from build123d import *

# Parameters (mm, degrees)
SKETCH_1_W          = 35
SKETCH_1_H          = 35
EXTRUDE_1_DEPTH     = 45
SKETCH_2_R          = 8.5
EXTRUDE_2_DEPTH     = 2.8
SKETCH_4_W          = 24
SKETCH_4_H          = 24
CUT_EXTRUDE_1_DEPTH = 40
SKETCH_5_R          = 3.25
CUT_EXTRUDE_2_DEPTH = 62.774509306


with BuildPart() as part:
    # 草图1 → 凸台-拉伸1 (new body)
    with BuildSketch(Plane(origin=(0, 0, 0), x_dir=(1, 0, 0), z_dir=(0, 1, 0))):
        Rectangle(SKETCH_1_W, SKETCH_1_H)
    extrude(amount=EXTRUDE_1_DEPTH)

    # 草图2 → 凸台-拉伸2 (add)
    with BuildSketch(Plane(origin=(0, 45, 0), x_dir=(1, 0, 0), z_dir=(0, 1, 0))):
        with Locations(Location((0, 0, 0), (0, 0, 270))):
            Circle(SKETCH_2_R)
    extrude(amount=EXTRUDE_2_DEPTH)

    # 草图4 → 切除-拉伸1 (cut)
    with BuildSketch(Plane.XZ):
        Rectangle(SKETCH_4_W, SKETCH_4_H)
    extrude(amount=-CUT_EXTRUDE_1_DEPTH, mode=Mode.SUBTRACT)

    # 草图5 → 切除-拉伸2 (cut, through all)
    with BuildSketch(Plane(origin=(17.5, 0, 0), x_dir=(0, 0, -1), z_dir=(1, 0, 0))):
        with Locations((0, 10.5)):
            Circle(SKETCH_5_R)
    extrude(amount=-CUT_EXTRUDE_2_DEPTH, mode=Mode.SUBTRACT)


solid = part.part
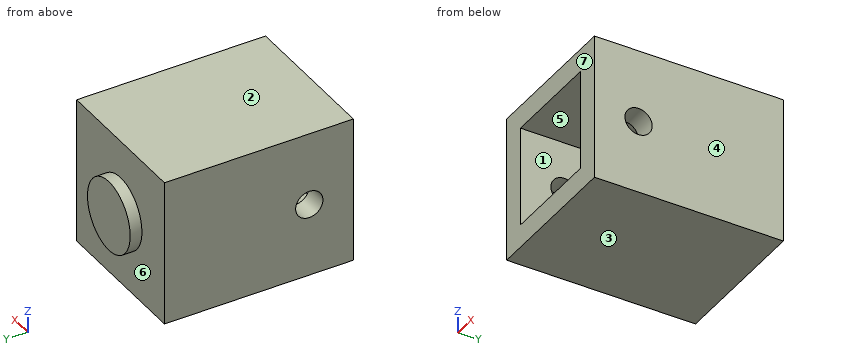
Read the model definition and answer for the solid it produces. Units are mm, in the model's axes. Face numbers are marked on the shaded views. A direction names the side the tool comes from. Coordinates: 2 decimals unless noted, no trailing zeros. Loops run counter-clockwise (first coordinate to the right, second up) from the corner with the lowest first, then second, coordinate; pieces in that order, holes last. Notation, with made-up numbers: (-31.5, 82) -> (13.5, 82) arc R7 ccw to (13.5, 95) -> close; hole circle Ø7 at (48, 54.25). An arc over 180 degrees is marked (long way). Answer in a Markdown table with one row per item.
Item 1: A cutting plane is placed at B-B on y = 10.5. Determine the outline of the cut face in (x, z), plus the area to 4 significant figures.
Returned:
| item | result |
|---|---|
| outline | (-17.5, -17.5) -> (17.5, -17.5) -> (17.5, -3.25) -> (12, -3.25) -> (12, -12) -> (-12, -12) -> (-12, -3.25) -> (-17.5, -3.25) -> close; (-17.5, 3.25) -> (-12, 3.25) -> (-12, 12) -> (12, 12) -> (12, 3.25) -> (17.5, 3.25) -> (17.5, 17.5) -> (-17.5, 17.5) -> close |
| area | 577.5 mm^2 |
Item 2: For a pull along Z with two mould halves and no side action, classify the marked faces 1, 2, 3 and 4 as released by +Z, released by -Z, zero draft, split by the parting line, or undercut.
Returned:
| item | result |
|---|---|
| face 1 | undercut |
| face 2 | released by +Z |
| face 3 | released by -Z |
| face 4 | zero draft |
Item 3: This flat-tipped pin is pushed along its axis until it touches: P1, Ø4, axis at x = 4.5, z = -6, coming from the -Y side. Where does it stop, or does it pass through?
Returned:
| item | result |
|---|---|
| P1 | stops at y = 40 |
Item 4: Straight lines are drawn through the part: line 1 along Y through (x, z) = (-13.7, 0); line 2 along X through (y, z) = (37, -5.5). For each, find the intervals that lie inside material, in ascending order. Write a range as [from, to].
Returned:
| item | result |
|---|---|
| line 1 | y = [0, 7.25], [13.75, 45] |
| line 2 | x = [-17.5, -12], [12, 17.5] |
Item 5: A cutting plane is placed at A-A on z = 0. Determine the outline of the cut face in (x, y), plus the area to 3 significant figures.
Returned:
| item | result |
|---|---|
| outline | (-17.5, 0) -> (-12, 0) -> (-12, 7.25) -> (-17.5, 7.25) -> close; (-17.5, 13.75) -> (-12, 13.75) -> (-12, 40) -> (12, 40) -> (12, 13.75) -> (17.5, 13.75) -> (17.5, 45) -> (8.5, 45) -> (8.5, 47.8) -> (-8.5, 47.8) -> (-8.5, 45) -> (-17.5, 45) -> close; (12, 0) -> (17.5, 0) -> (17.5, 7.25) -> (12, 7.25) -> close |
| area | 591 mm^2 |
Item 6: For the marked faces 5, 6 and 7, determine the directions among +Z, -Z, +X, -X, +Y, -Y from which every point of the face is accessible in a straight line to the end or side of a thin tool.
Returned:
| item | result |
|---|---|
| face 5 | -Y |
| face 6 | +Y |
| face 7 | +Z, -Z, +X, -X, -Y |
Item 7: A cutting plane is placed at D-D on y = 31. Determine the outline of the cut face in (x, z), plus the area to 3 significant figures.
Returned:
| item | result |
|---|---|
| outline | (-17.5, -17.5) -> (17.5, -17.5) -> (17.5, 17.5) -> (-17.5, 17.5) -> close; hole (-12, -12) -> (12, -12) -> (12, 12) -> (-12, 12) -> close |
| area | 649 mm^2 |
Item 8: A cutting plane is placed at C-C on x = 0. Determine the outline of the cut face in (y, z).
Returned:
| item | result |
|---|---|
| outline | (0, -17.5) -> (45, -17.5) -> (45, -8.5) -> (47.8, -8.5) -> (47.8, 8.5) -> (45, 8.5) -> (45, 17.5) -> (0, 17.5) -> (0, 12) -> (40, 12) -> (40, -12) -> (0, -12) -> close |
